Geometry check sheet. Reference: the model listing, model coordinates, mm. A direction names the side the tool comes from. Round coordinates to 2 decimals unless told otherwise and drop trailing zeros. Loops run counter-clockwise (first coordinate to the right, second up) from the corner with the lowest first, then second, coordinate; pieces in that order, holes last. Notation, with made-up numbers: M 53.5,74 L 66.5,74 A10 ccw 66.5,78 Z; hole C 76.25,-1 d6. An arc over 180 degrees is marked long. Write item = value, one per line.
from build123d import *

# Parameters (mm, degrees)
BOSS_EXTRUDE1_DEPTH                                 = 5
SKETCH4_W                                           = 10
SKETCH4_H                                           = 12
BOSS_EXTRUDE2_DEPTH                                 = 10
CBORE_FOR_M3_HEX_SOCKET_HEAD_CAP_SCREW1_D           = 3.2
CBORE_FOR_M3_HEX_SOCKET_HEAD_CAP_SCREW1_CBORE_D     = 6.5
CBORE_FOR_M3_HEX_SOCKET_HEAD_CAP_SCREW1_CBORE_DEPTH = 3
CHAMFER1_SIZE                                       = 6
BOSS_EXTRUDE3_START                                 = 3
SKETCH5_W                                           = 10
SKETCH5_H                                           = 10
SKETCH5_R                                           = 1.6
BOSS_EXTRUDE3_DEPTH                                 = 3
CUT_EXTRUDE1_DEPTH                                  = 4


with BuildPart() as part:
    # Sketch1 → Boss-Extrude1 (new, symmetric)
    with BuildSketch(Plane(origin=(0, 0, 0), x_dir=(1, 0, 0), z_dir=(0, 1, 0))):
        Polygon((0, 0), (-28, 0), (-28, 6), (-10, 6), (-10, 12), (0, 12), align=None)
    extrude(amount=BOSS_EXTRUDE1_DEPTH, both=True)

    # Sketch4 → Boss-Extrude2 (add)
    with BuildSketch(Plane.XZ.offset(5)):
        with Locations((-5, -6)):
            Rectangle(SKETCH4_W, SKETCH4_H)
    extrude(amount=BOSS_EXTRUDE2_DEPTH)

    # CBORE for M3 Hex Socket Head Cap Screw1 (through all)
    with Locations(Plane.XY):
        with Locations((-5, -10)):
            CounterBoreHole(CBORE_FOR_M3_HEX_SOCKET_HEAD_CAP_SCREW1_D / 2, CBORE_FOR_M3_HEX_SOCKET_HEAD_CAP_SCREW1_CBORE_D / 2, CBORE_FOR_M3_HEX_SOCKET_HEAD_CAP_SCREW1_CBORE_DEPTH)

    # Chamfer1
    chamfer1_edges = [part.edges().sort_by_distance(p)[0] for p in [
        (-5, 5, -12),
    ]]
    chamfer(chamfer1_edges, length=CHAMFER1_SIZE)

    # Sketch5 → Boss-Extrude3 (add)
    with BuildSketch(Plane(origin=(0, 0, -12), x_dir=(-1, 0, 0), z_dir=(0, 0, -1)).offset(BOSS_EXTRUDE3_START)):
        with Locations((5, -10)):
            Rectangle(SKETCH5_W, SKETCH5_H)
        with Locations(Location((5, -10, 0), (0, 0, 180))):
            Circle(SKETCH5_R, mode=Mode.SUBTRACT)
    extrude(amount=-BOSS_EXTRUDE3_DEPTH)

    # Sketch6 → Cut-Extrude1 (cut)
    with BuildSketch(Plane(origin=(0, 0, -15), x_dir=(-1, 0, 0), z_dir=(0, 0, -1))):
        Polygon((5, -13.233161507), (7.8, -11.616580754), (7.8, -8.383419246), (5, -6.766838493), (2.2, -8.383419246), (2.2, -11.616580754), align=None)
    extrude(amount=-CUT_EXTRUDE1_DEPTH, mode=Mode.SUBTRACT)


solid = part.part
(1) Sectioned sample at C-C on y = 3.25. Record the cut outline in (x, z), then the cut area to 4 significant figures.
Result set:
outline = M -28,-6 L -10,-6 L -10,-7.75 L 0,-7.75 L 0,0 L -28,0 Z
area = 185.5 mm2
(2) Sectioned sample at B-B on z = -9. Record the cut outline in (x, y).
Result set:
outline = M -10,-15 L 0,-15 L 0,2 L -10,2 Z; hole C -5,-10 d3.2
(3) Release check for a two-part mould opening along Y. For faces 6 (the flat face through (-14, 5, -3)), 7 (the flat face through (-6.38, -12.436, -13.028)), 8 (the flat face through (-10, -7, -8)), 9 (the cylindrical face through (-3.25, -7.26, -1.48)) record: released by +Y, released by -Y, zero draft, split by the parting line, or undercut.
Result set:
face_6 = released by +Y
face_7 = undercut
face_8 = zero draft
face_9 = undercut
(4) Sectioned sample at A-A on y = -10. Record the cut outline in (x, z), then the cut area to 3 significant figures.
Result set:
outline = M -10,-15 L -7.8,-15 L -7.8,-11 L -6.6,-11 L -6.6,-3 L -8.25,-3 L -8.25,0 L -10,0 Z; M -3.4,-11 L -2.2,-11 L -2.2,-15 L 0,-15 L 0,0 L -1.75,0 L -1.75,-3 L -3.4,-3 Z
area = 82.5 mm2
(5) Depth check by flat-ended pin: pin 1 Ø10 at (x, y) = (-10.5, -8.5) entering from +Z; pin 2 Ø3 at (x, y) = (-17.5, -2) entering from -Z; pin 3 Ø3 at (x, y) = (-5.5, -10.5) entering from +Z; pin 4 Ø6.5 at (x, z) = (-18.5, -3) entering from -Y. Enter the tip coordinate at first touch or a pass-through.
Result set:
pin_1 = 0
pin_2 = -6
pin_3 = -3
pin_4 = -5
(6) Sectioned sample at D-D on x = -22. Record the cut outline in (y, z), then the cut area to 3 significant figures.
Result set:
outline = M -5,-6 L 5,-6 L 5,0 L -5,0 Z
area = 60.0 mm2
(7) Material ranges on line 1 along Z through (x, y) = (-10.5, 3.75); line 2 along Z through (x, y) = (-9, -1); line 3 along X through (y, z) = (-8.5, -2.75), recorded low to high. Write a range as from..to.
Result set:
line_1 = -6..0
line_2 = -12..0
line_3 = -10..-7.88, -2.12..0
(8) Tool access check on faces 1 (the flat face through (-19, -5, -3)), 2 (the flat face through (-19, 0, -6)), 3 (the flat face through (-5, -5, -14)), 4 (the flat face through (-3.6, -11.4, -3)), 5 (the flat face through (-3.7, -11.4, -11)). Record the directions out of +Z, -Z, +X, -X, +Y, -Y that give a thin tool (end or side, any length) a straight path to the whole face; none if there is none.
Result set:
face_1 = +Z, -Z, -X, -Y
face_2 = -Z, -X, +Y, -Y
face_3 = -Z, +X, -X, +Y
face_4 = +Z
face_5 = -Z
